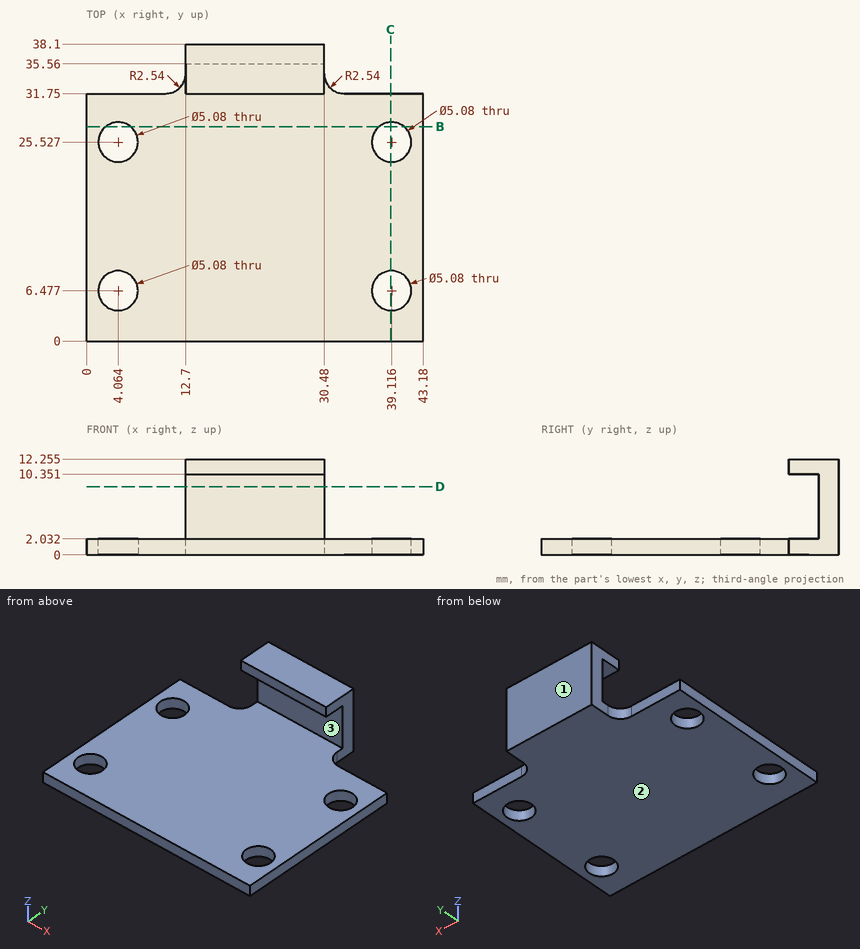
Here's the drawing with two shaded views (mm, measured from the low corner). I have some questions. Coordinates: 2 decimals unless noted, no trailing zeros. Order: outer loops, then holes, each group sorted by start corner. A loop starts at its lowest first (then second) coordinate and runs counter-clockwise, first axis right, second up. Notation, with made-up numbers: (38.5, 70.5) - (97.5, 70.5) arc R12 cw to (97.5, 87.5) - close; hole circle Ø8 at (57.25, 21). An arc over 180 degrees is marked (long way). Answer in a Markdown table with one row per item. Add a question column.
(1) If we section it at B-B, the plane y = 27.5: Please give me the cut outline in (x, z) (1 decimal).
(2) Will these pins go through, and if not, where does the flat tip stop? pin 1 (1.5 mm diameter, centred on x = 7.5, y = 20.5, fed in from +Z); pin 2 (2 mm diameter, centred on x = 37.5, z = 1, fed in from +Y); pin 3 (1.5 mm diameter, centred on x = 24, z = 11.5, fed in from -Y).
(3) If we section it at C-C, the plane x = 39: State how many separate pieces and enclosed holes the cut face has.
(4) If we mould it in two halves opening along Z, with no side actions, what happens to the marked faces 1, 2 and 3? For each: released by +Z, released by -Z, zero draft, split by the parting line, or undercut.
(5) I need wall thicknesses on L1, parallel to Z at x = 16, y = 10.5; L2, parallel to Y at x = 20, z = 3.25; L3, parallel to Y at x = 33, z = 1.5. Which ranges of each line are inside material? Lowest first, please.
(6) If we section it at D-D, the plane z = 8.75: Please give me the cut outline in (x, y).
Results are:
| question | item | result |
|---|---|---|
| 1 | outline | (0, 0) - (2.5, 0) - (2.5, 2) - (0, 2) - close; (5.7, 0) - (37.5, 0) - (37.5, 2) - (5.7, 2) - close; (40.7, 0) - (43.2, 0) - (43.2, 2) - (40.7, 2) - close |
| 2 | pin 1 | stops at z = 2.03 |
| 2 | pin 2 | stops at y = 31.75 |
| 2 | pin 3 | stops at y = 31.75 |
| 3 | separate pieces | 3 |
| 3 | enclosed holes | 0 |
| 4 | face 1 | zero draft |
| 4 | face 2 | released by -Z |
| 4 | face 3 | undercut |
| 5 | L1 | z = 0 to 2.03 |
| 5 | L2 | y = 35.56 to 38.1 |
| 5 | L3 | y = 0 to 31.75 |
| 6 | outline | (12.7, 35.56) - (30.48, 35.56) - (30.48, 38.1) - (12.7, 38.1) - close |
